from build123d import *

# Parameters (mm, degrees)
BOSS_EXTRUDE1_DEPTH = 20
SKETCH5_W           = 9
SKETCH5_H           = 1.454272164
CUT_EXTRUDE4_DEPTH  = 10
SKETCH6_R           = 0.5
CUT_EXTRUDE5_DEPTH  = 5


with BuildPart() as part:
    # Sketch1 → Boss-Extrude1 (new body)
    with BuildSketch(Plane.XY):
        with BuildLine():
            Line((0, 19.325625792), (0, -19.325625792))
            ThreePointArc((0, -19.325625792), (3.474436626, -26.903027896), (11.483404529, -29.214989321))
            Line((11.483404529, -29.214989321), (28.983404529, -26.589989321))
            ThreePointArc((28.983404529, -26.589989321), (35.077402104, -23.226189166), (37.5, -16.700625792))
            Line((37.5, -16.700625792), (37.5, 16.700625792))
            ThreePointArc((37.5, 16.700625792), (35.077402104, 23.226189166), (28.983404529, 26.589989321))
            Line((28.983404529, 26.589989321), (11.483404529, 29.214989321))
            ThreePointArc((11.483404529, 29.214989321), (3.474436626, 26.903027896), (0, 19.325625792))
        make_face()
    extrude(amount=BOSS_EXTRUDE1_DEPTH)

    # Sketch5 → Cut-Extrude4 (cut)
    with BuildSketch(Plane.ZY):
        with Locations((10, 16.569972364)):
            Rectangle(SKETCH5_W, SKETCH5_H)
    extrude(amount=-CUT_EXTRUDE4_DEPTH, mode=Mode.SUBTRACT)

    # Sketch6 → Cut-Extrude5 (cut)
    with BuildSketch(Plane.XZ.offset(-17.297108446)):
        with Locations((2.644871575, 10)):
            Circle(SKETCH6_R)
    extrude(amount=-CUT_EXTRUDE5_DEPTH, mode=Mode.SUBTRACT)


solid = part.part
Can you work these out from the model? Positions are in its coordinate system, mm. A direction names the side the tool comes from. Coordinates: 2 decimals unless noted, no trailing zeros. Loops run counter-clockwise (first coordinate to the right, second up) from the corner with the lowest first, then second, coordinate; pieces in that order, holes last. Notation, with made-up numbers: (-32, -31.75) - (12, -31.75) arc R30 cw to (12, 2.25) - close; hole circle Ø3 at (-3, -39). An arc over 180 degrees is marked (long way). Put each result on its own line as item: value. Start each with the question number.
Item 1: If we mould it in two halves opening along Y, with no side actions, what happens to faces 1 (the face through (5, 17, 14.5)), 2 (the face through (5, 15.843, 10)), 3 (the face through (20.356, 27.884, 9.86)), 4 (the face through (0, 0, 10))? For each: +Y half, -Y half, draft (parallel to the pull), parting line (faces both ways), or undercut.
Item 2: Which directions (+Z, -Z, +X, -X, +Y, -Y) give clear straight access to the entire face, cutting with the end or side of a thin tool? Please do faces 5 (the face through (37.5, 0, 10)), 6 (the face through (10, 17, 10)).
Item 3: Suppose I cut it at C-C (z = 1.5). Please give me the cut outline in (x, y), and give its area (3 significant figures).
Item 4: Suppose I cut it at A-A (z = 12.25). Please give me the cut outline in (x, y).
Item 5: Suppose I cut it at B-B (x = 30). Please give me the cut outline in (y, z), and give its area (3 significant figures).
Item 6: If I drill on line 1 along Y through (x, z) = (7.5, 10.5); line 2 along Y through (x, z) = (6, 10.25); line 3 along Y through (x, z) = (26, 17.25), over which ranges is the centre line in solid material (lowest first)?
Item 7: For pin 1 (7 mm diameter, centred on x = 4, z = 9.5, fed in from +Y); pin 2 (3 mm diameter, centred on x = 14, z = 11.5, fed in from -Y); pin 3 (2 mm diameter, centred on x = 12.5, z = 14.5, fed in from -Y), each with a flat end and sliding along its axis, tell me the tip position at first contact or that it passes through.
Here are the results:
1. face 1: undercut
1. face 2: undercut
1. face 3: +Y half
1. face 4: draft
2. face 5: +Z, -Z, +X, +Y, -Y
2. face 6: -X
3. outline: (0, -19.33) arc R10 ccw to (11.48, -29.21) - (28.98, -26.59) arc R10 ccw to (37.5, -16.7) - (37.5, 16.7) arc R10 ccw to (28.98, 26.59) - (11.48, 29.21) arc R10 ccw to (0, 19.33) - close
3. area: 2,020 mm²
4. outline: (0, -19.33) arc R10 ccw to (11.48, -29.21) - (28.98, -26.59) arc R10 ccw to (37.5, -16.7) - (37.5, 16.7) arc R10 ccw to (28.98, 26.59) - (11.48, 29.21) arc R10 ccw to (0, 19.33) - (0, 17.3) - (10, 17.3) - (10, 15.84) - (0, 15.84) - close
5. outline: (-26.38, 0) - (26.38, 0) - (26.38, 20) - (-26.38, 20) - close
5. area: 1,060 mm²
6. line 1: -29.01 to 15.84, 17.3 to 29.01
6. line 2: -28.49 to 15.84, 17.3 to 28.49
6. line 3: -27.04 to 27.04
7. pin 1: y = 29.01
7. pin 2: y = -29.06
7. pin 3: y = -29.21
